For this review, take the finished solid that the model builds, in its own axes (mm). A direction names the side the tool comes from. Round coordinates to 2 decimals unless told otherwise and drop trailing zeros. Write each loop counter-clockwise with the first axis right and the second up, starting at its lowest first coordinate (ties: lowest second). Pieces come first, ordered by that corner, then holes. Notation, with made-up numbers: (24, 36) - (50, 36) arc R25 cw to (50, 56) - close; hole circle Ø7 at (55.5, 53). An arc over 180 degrees is marked (long way). Answer in a Markdown table with one row per item. Add a question column.
from build123d import *

# Parameters (mm, degrees)
SKETCH1_W           = 22.225
SKETCH1_H           = 31.75
BOSS_EXTRUDE1_DEPTH = 6.35
FILLET1_R           = 3
BOSS_EXTRUDE2_DEPTH = 6.35
FILLET2_R           = 1
SKETCH3_R           = 1.5875
CUT_EXTRUDE1_DEPTH  = 16.35


with BuildPart() as part:
    # Sketch1 → Boss-Extrude1 (new body)
    with BuildSketch(Plane(origin=(0, 0, 0), x_dir=(1, 0, 0), z_dir=(0, 1, 0))):
        Rectangle(SKETCH1_W, SKETCH1_H)
    extrude(amount=BOSS_EXTRUDE1_DEPTH)

    # Fillet1
    fillet1_edges = [part.edges().sort_by_distance(p)[0] for p in [
        (11.1125, 3.175, 15.875),
        (-11.1125, 3.175, 15.875),
        (-11.1125, 3.175, -15.875),
        (11.1125, 3.175, -15.875),
    ]]
    fillet(fillet1_edges, radius=FILLET1_R)

    # Sketch2 → Boss-Extrude2 (add)
    with BuildSketch(Plane(origin=(0, 6.35, 0), x_dir=(1, 0, 0), z_dir=(0, 1, 0))):
        with BuildLine():
            Line((-17.4625, 28.575), (-14.058436423, -2.543223758))
            ThreePointArc((-14.058436423, -2.543223758), (-13.078889385, -4.450679351), (-11.076226608, -5.21699589))
            Line((-11.076226608, -5.21699589), (-6.223943536, -5.21699589))
            Line((-6.223943536, -5.21699589), (-6.223943536, -4.21699589))
            Line((-6.223943536, -4.21699589), (-11.076226608, -4.21699589))
            ThreePointArc((-11.076226608, -4.21699589), (-12.411335126, -3.706118197), (-13.064366485, -2.434481136))
            Line((-13.064366485, -2.434481136), (-16.468430062, 28.683742623))
            Line((-16.468430062, 28.683742623), (-17.4625, 28.575))
        make_face()
    extrude(amount=-BOSS_EXTRUDE2_DEPTH)

    # Fillet2
    fillet2_edges = [part.edges().sort_by_distance(p)[0] for p in [
        (-16.965465031, 6.35, -28.629371311),
        (-16.965465031, 0, -28.629371311),
    ]]
    fillet(fillet2_edges, radius=FILLET2_R)

    # Sketch3 → Cut-Extrude1 (cut)
    with BuildSketch(Plane(origin=(0, 6.35, 0), x_dir=(1, 0, 0), z_dir=(0, 1, 0))):
        with Locations((7.756160145, 12.478354906)):
            Circle(SKETCH3_R)
        with Locations((-7.930929808, -12.598511213)):
            Circle(SKETCH3_R)
    extrude(amount=-CUT_EXTRUDE1_DEPTH, mode=Mode.SUBTRACT)


solid = part.part
Q1. Tool access review of faces 4 (the face through (-11.112, 3, 9)), 5 (the face through (0, 3, -15.875)), 6 (the face through (-14.743, 3.219, -12.907)), 7 (the face through (-7.08, 3.22, 11.26)): name each direction out of +Z, -Z, +X, -X, +Y, -Y from which nothing blocks a thin tool from reaching the whole face with its end or side.
Q2. Draft analysis for pull direction X (two halves, no side actions). For faces 1 (the face through (10.26, 3.22, -14.97)), 2 (the face through (-16.941, 0.301, -28.345)), 3 (the face through (-11.112, 3, -4)), state which applies: released by +X, released by -X, zero draft, split by the parting line, or undercut.
Q3. Add section B-B on y = 4. State the section outline as (x, z) points (1 decimal).
Q4. Add section C-C on z = -8. State the section outline as (x, y) points, then the cut area to 3 significant figures.
Q5. Insertion check: pin 1 Ø3 at (y, z) = (2, -2) entering from -X; pin 2 Ø3 at (y, z) = (1.5, 9.5) entering from -X; pin 3 Ø1.5 at (y, z) = (2, -2) entering from -X. Each pin has a flat end and moves straight along its axis. Give the tip position at first contact, or say it passes through.
Q6. Add section A-A on z = -15. State the section outline as (x, y) points.
Q7. To check wall thickness, follow probe 1 along X at (y, z) = (3.75, -13.5); probe 2 along X at (y, z) = (1.5, 12.5); probe 3 along Z at (x, y) = (-1, 2) (3 decimals). State the ranges of each line that lie inside material, in increasing order.
Q8. Add section D-D on x = 4. State the section outline as (y, z) points (3 decimals), then the cut area to 3 significant figures.
Answer sheet:
| question | item | result |
|---|---|---|
| 1 | face 4 | +Z, -X, +Y, -Y |
| 1 | face 5 | -Z, +X, +Y, -Y |
| 1 | face 6 | -Z, +Y, -Y |
| 1 | face 7 | +Y, -Y |
| 2 | face 1 | released by +X |
| 2 | face 2 | released by -X |
| 2 | face 3 | undercut |
| 3 | outline | (-17.5, -28.6) - (-16.5, -28.7) - (-13.1, 2.4) arc R2 cw to (-11.1, 4.2) - (-11.1, -12.9) arc R3 ccw to (-8.1, -15.9) - (8.1, -15.9) arc R3 ccw to (11.1, -12.9) - (11.1, 12.9) arc R3 ccw to (8.1, 15.9) - (-8.1, 15.9) arc R3 ccw to (-11.1, 12.9) - (-11.1, 5.2) arc R3 ccw to (-14.1, 2.5) - close; hole circle Ø3.2 at (-7.9, 12.6); hole circle Ø3.2 at (7.8, -12.5) |
| 4 | outline | (-15.21, 0) - (-14.21, 0) - (-14.21, 6.35) - (-15.21, 6.35) - close; (-11.11, 0) - (11.11, 0) - (11.11, 6.35) - (-11.11, 6.35) - close |
| 4 | area | 148 mm² |
| 5 | pin 1 | stops at x = -14.72 |
| 5 | pin 2 | stops at x = -11.11 |
| 5 | pin 3 | stops at x = -14.64 |
| 6 | outline | (-15.98, 0) - (-14.97, 0) - (-14.97, 6.35) - (-15.98, 6.35) - close; (-10.23, 0) - (10.23, 0) - (10.23, 6.35) - (-10.23, 6.35) - close |
| 7 | probe 1 | x = -15.81 to -14.81, -11.05 to 6.54, 8.97 to 11.05 |
| 7 | probe 2 | x = -11.11 to -9.52, -6.35 to 11.11 |
| 7 | probe 3 | z = -15.875 to 15.875 |
| 8 | outline | (0, -15.875) - (6.35, -15.875) - (6.35, 15.875) - (0, 15.875) - close |
| 8 | area | 202 mm² |
